```python
from build123d import *

# Parameters (mm, degrees)
F1_DEPTH = 25
F3_D     = 10
F4_D     = 10
F5_R     = 5


with BuildPart() as f1:
    # F0 (on Front) → F1 (new body)
    with BuildSketch(Plane.XZ):
        with BuildLine():
            Line((-29.814812, 8), (-29.814812, 0))
            Line((-29.814812, 0), (40.185188, 0))
            Line((40.185188, 0), (40.185188, 8))
            Line((40.185188, 8), (19.814818, 8))
            Line((19.814818, 8), (19.814818, 28))
            Line((19.814818, 28), (15.746092, 28))
            ThreePointArc((15.746092, 28), (5.185188, 17.439096), (-5.375716, 28))
            Line((-5.375716, 28), (-9.444442, 28))
            Line((-9.444442, 28), (-9.444442, 8))
            Line((-9.444442, 8), (-29.814812, 8))
        make_face()
    extrude(amount=F1_DEPTH)

    # F3 (through all)
    with Locations(Plane.XY.offset(8)):
        with Locations((-19.629627, -12.5)):
            Hole(F3_D / 2)

    # F4 (through all)
    with Locations(Plane.XY.offset(8)):
        with Locations((30.000003, -12.5)):
            Hole(F4_D / 2)

    # F5
    f5_edges = [f1.edges().sort_by_distance(p)[0] for p in [
        (-9.444442, -12.5, 8),
        (19.814818, -12.5, 8),
    ]]
    fillet(f5_edges, radius=F5_R)


solid = f1.part
```
Check sheet for the modelled part. Datum: model origin and axes. Units: mm. A direction names the side the tool comes from. Round coordinates to 2 decimals unless told otherwise and drop trailing zeros. Order: outer loops, then holes, each group sorted by start corner. A loop starts at its lowest first (then second) coordinate and runs counter-clockwise, first axis right, second up. Notation, with made-up numbers: (47, -13.75) - (94, -13.75) arc R20 cw to (94, -3.75) - close; hole circle Ø7 at (-31.75, -37). An arc over 180 degrees is marked (long way). Answer as CSV lines item,"result". Start each with the question number.
1) Draft check along Y on faces 1 (the face through (5, 0, 8)), 2 (the face through (34.995, -12.28, 3.944)), 3 (the face through (5, -25, 8)), 4 (the face through (-25, -12, 8)). Enter one of: +Y half, -Y half, draft (parallel to the pull), parting line (faces both ways), or undercut.
2) Tool access check on faces 5 (the face through (-9.444, -12, 21)), 6 (the face through (-24.4, -11, 3.9)), 7 (the face through (19.815, -12, 20)). Record the directions out of +Z, -Z, +X, -X, +Y, -Y that give a thin tool (end or side, any length) a straight path to the whole face; none if there is none.
3) Section check A-A (y = -12.5). Record the cut outline in (x, z).
4) Scan lines: probe 1 along X at (y, z) = (-16, 6.75); probe 2 along Z at (x, y) = (25.5, -3.5); probe 3 along X at (y, z) = (-2, 22.25). Record each from-to range of solid material in increasing order.
5) Section check D-D (z = 21). Record the cut outline in (x, y).
6) Section check B-B (z = 2.75). Record the cut outline in (x, y).
7) Section check C-C (x = 29). Record the cut outline in (y, z).
8) Depth check by flat-ended pin: pin 1 (7.5 mm diameter, centred on y = -18.5, z = 21.5, fed in from -X); pin 2 (1.5 mm diameter, centred on x = -16, y = -16, fed in from +Z); pin 3 (3 mm diameter, centred on x = 19.5, y = -6, fed in from -Z); pin 4 (3 mm diameter, centred on y = -18, z = 11, fed in from +X). Enter the tip coordinate at first touch or a pass-through.
Determined:
1,face 1,"+Y half"
1,face 2,"undercut"
1,face 3,"-Y half"
1,face 4,"draft"
2,face 5,"+Z, -X, +Y, -Y"
2,face 6,"+Z, -Z"
2,face 7,"+Z, +X, +Y, -Y"
3,outline,"(-29.81, 0) - (-24.63, 0) - (-24.63, 8) - (-29.81, 8) - close; (-14.63, 0) - (25, 0) - (25, 8) - (24.81, 8) arc R5 cw to (19.81, 13) - (19.81, 28) - (15.75, 28) arc R10.56 cw to (-5.38, 28) - (-9.44, 28) - (-9.44, 13) arc R5 cw to (-14.44, 8) - (-14.63, 8) - close; (35, 0) - (40.19, 0) - (40.19, 8) - (35, 8) - close"
4,probe 1,"-29.81 to -23.2, -16.06 to 26.43, 33.57 to 40.19"
4,probe 2,"0 to 8"
4,probe 3,"-9.44 to -3.67, 14.04 to 19.81"
5,outline,"(-9.44, -25) - (-2.72, -25) - (-2.72, 0) - (-9.44, 0) - close; (13.09, -25) - (19.81, -25) - (19.81, 0) - (13.09, 0) - close"
6,outline,"(-29.81, -25) - (40.19, -25) - (40.19, 0) - (-29.81, 0) - close; hole circle Ø10 at (-19.63, -12.5); hole circle Ø10 at (30, -12.5)"
7,outline,"(-25, 0) - (-17.4, 0) - (-17.4, 8) - (-25, 8) - close; (-7.6, 0) - (0, 0) - (0, 8) - (-7.6, 8) - close"
8,pin 1,"x = -9.44"
8,pin 2,"z = 8"
8,pin 3,"z = 0"
8,pin 4,"x = 21.24"
